from build123d import *

# Parameters (mm, degrees)
F0_W      = 152.4
F0_H      = 71.12
F1_DEPTH  = 44.45
F2_T      = -2.54
F3_W      = 2.54
F3_H      = 63.5
F4_DEPTH  = 83.82
F5_W      = 147.32
F5_H      = 2.54
F5_W_2    = 149.86
F6_DEPTH  = 2.54
F7_W      = 147.32
F7_H      = 2.54
F7_W_2    = 149.86
F8_DEPTH  = 2.54
F9_W      = 78.74
F9_H      = 2.54
F10_DEPTH = 2.54
F11_W     = 3.556
F11_H     = 2.54
F12_DEPTH = 127
F13_R     = 2.53999
F14_W     = 12.7
F14_H     = 25.4
F15_DEPTH = 254


# Not quite as in the source:
# - a fillet or chamfer is up to 0.001 mm smaller than in the source, because OpenCascade refuses the exact size


with BuildPart() as f1:
    # F0 (on Right) → F1 (new body, symmetric)
    with BuildSketch(Plane.YZ):
        Rectangle(F0_W, F0_H)
    extrude(amount=F1_DEPTH, both=True)

    # F2
    f2_openings = [f1.faces().sort_by_distance(p)[0] for p in [
        (0, 0, 35.56),
        (0, 76.2, 0),
    ]]
    offset(amount=F2_T, openings=f2_openings)

    # F3 (on face) → F4 (join, through all)
    with BuildSketch(Plane.YZ.offset(-41.91)):
        with Locations((74.93, -1.27)):
            Rectangle(F3_W, F3_H)
    extrude(amount=F4_DEPTH)

    # F5 (on face) → F6 (join)
    with BuildSketch(Plane(origin=(41.91, 0, 0), x_dir=(0, -1, 0), z_dir=(-1, 0, 0))):
        with Locations((0, 29.21)):
            Rectangle(F5_W, F5_H)
        with Locations((-1.27, 34.29)):
            Rectangle(F5_W_2, F5_H)
    extrude(amount=F6_DEPTH)

    # F7 (on face) → F8 (join)
    with BuildSketch(Plane.YZ.offset(-41.91)):
        with Locations((0, 29.21)):
            Rectangle(F7_W, F7_H)
        with Locations((1.27, 34.29)):
            Rectangle(F7_W_2, F7_H)
    extrude(amount=F8_DEPTH)

    # F9 (on face) → F10 (join)
    with BuildSketch(Plane(origin=(0, -73.66, 0), x_dir=(-1, 0, 0), z_dir=(0, 1, 0))):
        with Locations((0, 34.29)):
            Rectangle(F9_W, F9_H)
        with Locations((0, 29.21)):
            Rectangle(F9_W, F9_H)
    extrude(amount=F10_DEPTH)

    # F11 (on face) → F12 (cut, symmetric)
    with BuildSketch(Plane.YZ.offset(-41.91)):
        Polygon((-73.66, -5.08), (-73.66, -27.94), (-69.3801, -27.94), (-69.3801, -25.4), (-65.8241, -25.4), (-65.8241, -27.94), (-61.5442, -27.94), (-61.5442, -5.08), align=None)
        with Locations((-67.6021, -26.67)):
            Rectangle(F11_W, F11_H)
        with Locations((-67.6021, -29.21)):
            Rectangle(F11_W, F11_H)
    extrude(amount=F12_DEPTH, both=True, mode=Mode.SUBTRACT)

    # F13 (radius 2.54 in the source; OpenCascade refuses exactly that, so slightly less here)
    f13_edges = [f1.edges().sort_by_distance(p)[0] for p in [
        (0, -76.2, -35.56),
        (-44.45, 0, -35.56),
        (44.45, 0, -35.56),
        (44.45, -76.2, 0),
        (-44.45, -76.2, 0),
        (0, 76.2, -35.56),
        (44.45, 76.2, 0),
        (-44.45, 76.2, 0),
        (0, -76.2, 35.56),
        (44.45, 0, 35.56),
        (-44.45, 0, 35.56),
    ]]
    fillet(f13_edges, radius=F13_R)

    # F14 (on face) → F15 (cut)
    with BuildSketch(Plane.YZ.offset(44.45)):
        with Locations((-39.37, 12.7)):
            Rectangle(F14_W, F14_H)
        with Locations((-16.51, 12.7)):
            Rectangle(F14_W, F14_H)
        with Locations((6.35, 12.7)):
            Rectangle(F14_W, F14_H)
        with Locations((29.21, 12.7)):
            Rectangle(F14_W, F14_H)
        with Locations((52.07, 12.7)):
            Rectangle(F14_W, F14_H)
    extrude(amount=-F15_DEPTH, mode=Mode.SUBTRACT)


solid = f1.part
The model under review builds one solid part; all positions refer to its coordinate system, in mm. A direction names the side the tool comes from. Round coordinates to 2 decimals unless told otherwise and drop trailing zeros. Order: outer loops, then holes, each group sorted by start corner. A loop starts at its lowest first (then second) coordinate and runs counter-clockwise, first axis right, second up. Notation, with made-up numbers: (45, 25.5) -> (91, 25.5) arc R6 ccw to (91, 30.5) -> close; hole circle Ø2 at (-23, -16). An arc over 180 degrees is marked (long way). Write item = value, one per line. Start each with the question number.
Item 1: Clearance check with flat-ended pins moving along their axes: pin 1 Ø2 at (x, y) = (-43.5, 7) entering from -Z; pin 2 Ø5 at (y, z) = (6, 3.5) entering from +X; pin 3 Ø0.8 at (x, z) = (-11, 34.5) entering from +Y; pin 4 Ø0.8 at (x, z) = (-43.5, -19) entering from -Y. State where each tip first meets the part, or that it passes through.
Item 2: Mouldability with a two-part tool opening along Z and no side actions: class faces 4 (the face through (-44.45, -1, 0)), 5 (the face through (40, -22, 27.94)), 6 (the face through (1, -1, -35.56)) as released by +Z, released by -Z, zero draft, split by the parting line, or undercut.
Item 3: For line 1 along Y through (x, z) = (7, -21); line 2 along X through (y, z) = (-47, -1), list the stretches that pass through material, from the lowest coordinate up.
Item 4: For faces 1 (the face through (1, -73.66, -2)), 2 (the face through (-40, -21, 35.56)), 3 (the face through (41, -21, 33.02)), list the 3-axis set-ups (+Z, -Z, +X, -X, +Y, -Y) from which the entire face can be reached by the end or side of a thin tool; tool diameter is ignored.
Item 5: Consider section D-D on y = -49. Write out the cut boundary in (x, z), plus the area to 3 significant figures.
Item 6: Consider section B-B on y = 29. Count the separate pieces of the cut face and the enclosed holes in it, plus the area to 3 significant figures.
Item 7: Consider section C-C on x = -23.5. Write out the cut boundary in (y, z).
Conclusion:
q1.pin_1 = -35.49
q1.pin_2 = through
q1.pin_3 = -71.12
q1.pin_4 = -75.9
q2.face_4 = zero draft
q2.face_5 = undercut
q2.face_6 = released by -Z
q3.line_1 = -76.2 to -73.66, 73.66 to 76.2
q3.line_2 = -44.45 to -41.91, 41.91 to 44.45
q4.face_1 = none
q4.face_2 = +Z, +X, -X, +Y, -Y
q4.face_3 = +Y
q5.outline = (-44.45, -33.02) arc R2.54 ccw to (-41.91, -35.56) -> (41.91, -35.56) arc R2.54 ccw to (44.45, -33.02) -> (44.45, 33.02) arc R2.54 ccw to (41.91, 35.56) -> (39.37, 35.56) -> (39.37, 33.02) -> (41.91, 33.02) -> (41.91, 30.48) -> (39.37, 30.48) -> (39.37, 27.94) -> (41.91, 27.94) -> (41.91, -33.02) -> (-41.91, -33.02) -> (-41.91, 27.94) -> (-39.37, 27.94) -> (-39.37, 30.48) -> (-41.91, 30.48) -> (-41.91, 33.02) -> (-39.37, 33.02) -> (-39.37, 35.56) -> (-41.91, 35.56) arc R2.54 ccw to (-44.45, 33.02) -> close
q5.area = 594 mm2
q6.separate_pieces = 3
q6.enclosed_holes = 0
q6.area = 465 mm2
q7.outline = (-76.2, -33.02) arc R2.54 ccw to (-73.66, -35.56) -> (73.66, -35.56) arc R2.54 ccw to (76.2, -33.02) -> (76.2, 30.48) -> (73.66, 30.48) -> (73.66, -33.02) -> (-73.66, -33.02) -> (-73.66, 27.94) -> (-71.12, 27.94) -> (-71.12, 30.48) -> (-73.66, 30.48) -> (-73.66, 33.02) -> (-71.12, 33.02) -> (-71.12, 35.56) -> (-73.66, 35.56) arc R2.54 ccw to (-76.2, 33.02) -> close
